Source: CAD feature listing. Evaluate the final solid. Frame: model axes, mm. A direction names the side the tool comes from. Give positions to 0.01 mm unless a question says otherwise; leave off trailing zeros. Order: outer loops, then holes, each group sorted by start corner. A loop starts at its lowest first (then second) coordinate and runs counter-clockwise, first axis right, second up. Notation, with made-up numbers: M -13.5,-23 L 23.5,-23 A8 cw 23.5,-16 Z; hole C -1.75,5.5 d11. An arc over 180 degrees is marked long. Return JSON: item names as keys, results as strings.
from build123d import *

# Parameters (mm, degrees)
SKETCH1_R           = 1.75
BOSS_EXTRUDE1_DEPTH = 2.5
SKETCH2_R           = 6
BOSS_EXTRUDE2_DEPTH = 5.5
SKETCH3_R           = 3
BOSS_EXTRUDE3_DEPTH = 15
CHAMFER1_SIZE       = 0.7
SKETCH4_W           = 12
SKETCH4_H           = 2.8
CUT_EXTRUDE1_DEPTH  = 66.015382795
CHAMFER2_SIZE       = 0.5
SKETCH5_R           = 21
BOSS_EXTRUDE4_DEPTH = 31
FILLET1_R           = 2
SKETCH6_R           = 20
BOSS_EXTRUDE5_DEPTH = 35
FILLET2_R           = 2
FILLET3_R           = 1


# Some blends are built 0.0001 mm under size
with BuildPart() as part:
    # Sketch1 → Boss-Extrude1 (new body)
    with BuildSketch(Plane.XY):
        with BuildLine():
            Line((3.5, 0), (39.5, 0))
            ThreePointArc((39.5, 0), (41.974873734, -1.025126266), (43, -3.5))
            Line((43, -3.5), (43, -39.5))
            ThreePointArc((43, -39.5), (41.974873734, -41.974873734), (39.5, -43))
            Line((39.5, -43), (3.5, -43))
            ThreePointArc((3.5, -43), (1.025126266, -41.974873734), (0, -39.5))
            Line((0, -39.5), (0, -3.5))
            ThreePointArc((0, -3.5), (1.025126266, -1.025126266), (3.5, 0))
        make_face()
        with Locations((3.5, -3.5)):
            Circle(SKETCH1_R, mode=Mode.SUBTRACT)
        with Locations((39.5, -3.5)):
            Circle(SKETCH1_R, mode=Mode.SUBTRACT)
        with Locations((3.5, -39.5)):
            Circle(SKETCH1_R, mode=Mode.SUBTRACT)
        with Locations((39.5, -39.5)):
            Circle(SKETCH1_R, mode=Mode.SUBTRACT)
    extrude(amount=BOSS_EXTRUDE1_DEPTH)

    # Sketch2 → Boss-Extrude2 (add)
    with BuildSketch(Plane.XY.offset(2.5)):
        with Locations((21.5, -14.5)):
            Circle(SKETCH2_R)
    extrude(amount=BOSS_EXTRUDE2_DEPTH)

    # Sketch3 → Boss-Extrude3 (add)
    with BuildSketch(Plane.XY.offset(8)):
        with Locations((21.5, -14.5)):
            Circle(SKETCH3_R)
    extrude(amount=BOSS_EXTRUDE3_DEPTH)

    # Chamfer1
    chamfer1_edges = [part.edges().sort_by_distance(p)[0] for p in [
        (15.5, -14.5, 8),
    ]]
    chamfer(chamfer1_edges, length=CHAMFER1_SIZE)

    # Sketch4 → Cut-Extrude1 (cut, through all)
    with BuildSketch(Plane(origin=(43, 0, 0), x_dir=(0, 0, -1), z_dir=(1, 0, 0))):
        with Locations((-17, -10.6)):
            Rectangle(SKETCH4_W, SKETCH4_H)
    extrude(amount=-CUT_EXTRUDE1_DEPTH, mode=Mode.SUBTRACT)

    # Chamfer2
    chamfer2_edges = [part.edges().sort_by_distance(p)[0] for p in [
        (20.081362835, -17.143382037, 23),
    ]]
    chamfer(chamfer2_edges, length=CHAMFER2_SIZE - 0.0001)  # a hair under: the kernel refuses the full size

    # Sketch5 → Boss-Extrude4 (add)
    with BuildSketch(Plane(origin=(0, 0, 0), x_dir=(-1, 0, 0), z_dir=(0, 0, -1))):
        with Locations(Location((-21.5, -21.5, 0), (0, 0, 180))):
            Circle(SKETCH5_R)
    extrude(amount=BOSS_EXTRUDE4_DEPTH)

    # Fillet1
    fillet1_edges = [part.edges().sort_by_distance(p)[0] for p in [
        (0.5, -21.5, -31),
    ]]
    fillet(fillet1_edges, radius=FILLET1_R)

    # Sketch6 → Boss-Extrude5 (add)
    with BuildSketch(Plane(origin=(0, 0, -31), x_dir=(-1, 0, 0), z_dir=(0, 0, -1))):
        with Locations((-21.5, -21.5)):
            Circle(SKETCH6_R)
    extrude(amount=BOSS_EXTRUDE5_DEPTH)

    # Fillet2
    # the kernel refuses this fillet: 2 mm, written as the material it takes off along each edge
    with BuildSketch(Plane(origin=(21.5, -21.5, -31), x_dir=(-1, 0, 0), z_dir=(0, -1, 0))) as fillet2_piece_1:
        with BuildLine():
            CenterArc((18, 1.732050808), FILLET2_R, 300, 60)
            Line((19, 0), (20, 0))
            Line((20, 0), (20, 1.732050808))
        make_face()
    revolve(axis=Axis((21.5, -21.5, -31), (0, 0, -1)), mode=Mode.SUBTRACT)

    # Fillet3
    fillet3_edges = [part.edges().sort_by_distance(p)[0] for p in [
        (41.5, -21.5, -66),
    ]]
    fillet(fillet3_edges, radius=FILLET3_R)

    # Sketch7 → Cut-Revolve1 (revolve, cut)
    with BuildSketch(Plane(origin=(21.5, 0, 0), x_dir=(0, 0, -1), z_dir=(1, 0, 0)), mode=Mode.PRIVATE) as cut_revolve1_sk:
        with BuildLine():
            Line((-2.5, -1.5), (-1.5, -1.5))
            add(Edge.make_bspline(
                [(-2.5, -0.5), (-2.2, -1.2), (-1.5, -1.5)],
                knots=[0, 0, 0, 1, 1, 1], degree=2))
            Line((-2.5, -0.5), (-2.5, -1.5))
        make_face()
    revolve(cut_revolve1_sk.sketch.rotate(Axis((21.5, -21.5, -66), (0, 0, 1)), 90), axis=Axis((21.5, -21.5, -66), (0, 0, 1)), mode=Mode.SUBTRACT)


solid = part.part
1. Set-up query: faces 5 (the face through (22, -12, 17)), 6 (the face through (20.85, -17.43, 15.15)), 7 (the face through (21, 0, 1)), 8 (the face through (2.424, -15.493, -48.64)). Return all of +Z, -Z, +X, -X, +Y, -Y with unobstructed straight access to the full face (end or side cutting, diameter ignored); none if empty.
Evaluation:
{"face 5": "+Z, +X, -X, +Y", "face 6": "+Z", "face 7": "+Z, -Z, +X, -X, +Y", "face 8": "-Z"}
2. Ray query, probe 1 along Y at (x, z) = (3.5, 1.25); probe 2 along X at (y, z) = (-39, 1); probe 3 along Z at (x, y) = (33.5, -12.5). Return the intervals inside material, ascending.
Evaluation:
{"probe 1": "y = -43 to -41.25, -37.75 to -5.25, -1.75 to 0", "probe 2": "x = 0 to 1.82, 5.18 to 37.82, 41.18 to 43", "probe 3": "z = -66 to 2.5"}
3. Section query A-A (z = -53.5). Return loops of the section in (x, y).
Evaluation:
{"outline": "C 21.5,-21.5 d40"}
4. Draft query along Y for faces 1 (the face through (25.836, -1.976, 1.993)), 2 (the face through (6.02, -35.69, -14.3)), 3 (the face through (41.117, -4.17, 1.232)), 4 (the face through (1, -1.05, 1.23)). Return one class per face: pulls with the +Y half, pulls with the -Y half, needs draft (parallel to the pull), parting line crosses it, or undercut.
Evaluation:
{"face 1": "undercut", "face 2": "parting line crosses it", "face 3": "undercut", "face 4": "pulls with the +Y half"}
5. First-contact query: pin 1 (5.5 mm diameter, centred on x = 39.5, y = -39.5, fed in from +Z); pin 2 (8 mm diameter, centred on x = 21.5, z = -43, fed in from +Y); pin 3 (1.5 mm diameter, centred on x = 35, z = -13.5, fed in from +Y); pin 4 (2 mm diameter, centred on x = 3.5, y = -39.5, fed in from +Z). Flat tips, straight axial feed; report the tip coordinate or a pass-through.
Evaluation:
{"pin 1": "stops at z = 2.5", "pin 2": "stops at y = -1.5", "pin 3": "stops at y = -4.81", "pin 4": "passes through"}
